Input: dimensioned drawing with shaded views. Units: mm. Origin: part minimum x, y, z. A direction names the side the tool comes from. Round coordinates to 2 decimals unless told otherwise and drop trailing zeros. Order: outer loops, then holes, each group sorted by start corner. A loop starts at its lowest first (then second) coordinate and runs counter-clockwise, first axis right, second up.
Item 1: Cut plane D-D on x = 40. Output: boundary loops of the cut face in (y, z) (1 decimal).
Item 2: Mould query, pull axis Y, two halves, no side actions, for the marked faces 4, 5 and 6. Classes: released by +Y, released by -Y, zero draft, split by the parting line, or undercut.
Item 3: First-contact query: pin 1 (19 mm diameter, centred on x = 72, y = 37.5, fed in from +Z); pin 2 (12 mm diameter, centred on y = 21.5, z = 37, fed in from +X); pin 3 (10.5 mm diameter, centred on y = 42, z = 7.5, fed in from +X). Flat tips, straight axial feed; report the tip coordinate or a pass-through.
Item 4: Line query: L1, parallel to Y at x = 79, z = 16 (1 decimal); L2, parallel to X at y = 9, z = 52.5; L3, parallel to Y at x = 44.5, z = 43 (1 decimal). Output: solid intervals per line, ascending.
Item 5: Cut plane B-B on y = 55. Output: boundary loops of the cut face in (x, z).
Item 6: Reachability of the marked faces 1, 2 and 3 from +Z, -Z, +X, -X, +Y, -Y: full face, straight path, thin tool, end or side. Return the list, or none.
Item 7: Cut plane A-A on x = 83.5. Output: boundary loops of the cut face in (y, z) (1 decimal), then the cut area to 3 significant figures.
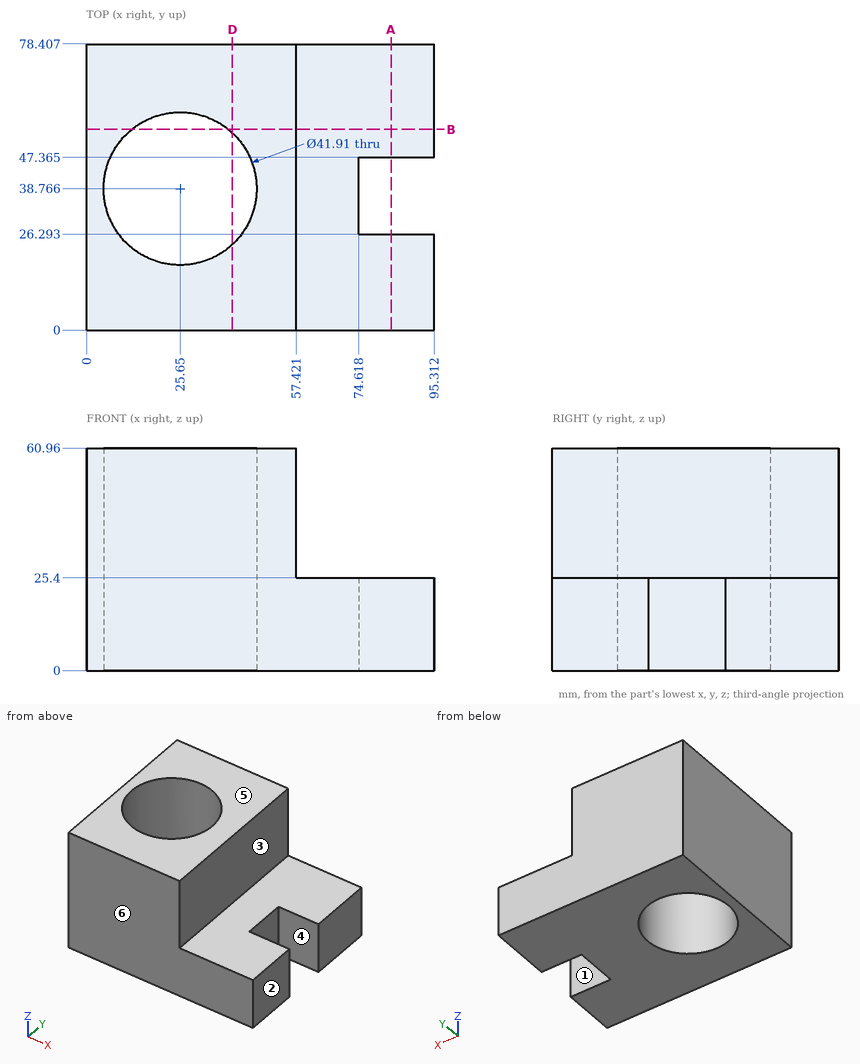
From the geometry:
1. outline: (0, 0) - (23.5, 0) - (23.5, 61) - (0, 61) - close; (54, 0) - (78.4, 0) - (78.4, 61) - (54, 61) - close
2. face 4: undercut
2. face 5: zero draft
2. face 6: released by -Y
3. pin 1: stops at z = 25.4
3. pin 2: stops at x = 57.42
3. pin 3: stops at x = 74.62
4. L1: y = 0 to 26.3, 47.4 to 78.4
4. L2: x = 0 to 57.42
4. L3: y = 0 to 29.6, 47.9 to 78.4
5. outline: (0, 0) - (12.4, 0) - (12.4, 60.96) - (0, 60.96) - close; (38.9, 0) - (95.31, 0) - (95.31, 25.4) - (57.42, 25.4) - (57.42, 60.96) - (38.9, 60.96) - close
6. face 1: +Z, -Z, +X
6. face 2: +Z, -Z, +X, +Y, -Y
6. face 3: +Z, +X, +Y, -Y
7. outline: (0, 0) - (26.3, 0) - (26.3, 25.4) - (0, 25.4) - close; (47.4, 0) - (78.4, 0) - (78.4, 25.4) - (47.4, 25.4) - close
7. area: 1,460 mm2
